```python
from build123d import *

# Parameters (mm, degrees)
F1_DEPTH = 304.8
F2_SIZE  = 50.79999
F3_SIZE  = 50.79999


# Not quite as in the source:
# - a fillet or chamfer is up to 0.001 mm smaller than in the source, because OpenCascade refuses the exact size


with BuildPart() as f1:
    # F0 (on Front) → F1 (new body, symmetric)
    with BuildSketch(Plane.XZ):
        Polygon((76.2, 3.175), (76.2, 0), (127, 0), (127, 50.8), (123.825, 50.8), (123.825, 3.175), align=None)
    extrude(amount=F1_DEPTH, both=True)

    # F2 (size 50.8 in the source; OpenCascade refuses exactly that, so slightly less here)
    f2_edges = [f1.edges().sort_by_distance(p)[0] for p in [
        (76.2, -304.8, 1.5875),
    ]]
    chamfer(f2_edges, length=F2_SIZE)

    # F3 (size 50.8 in the source; OpenCascade refuses exactly that, so slightly less here)
    f3_edges = [f1.edges().sort_by_distance(p)[0] for p in [
        (76.2, 304.8, 1.5875),
    ]]
    chamfer(f3_edges, length=F3_SIZE)


solid = f1.part
```
Could you check a few things on this model? Use its own coordinates, in mm. A direction names the side the tool comes from. Coordinates: 2 decimals unless noted, no trailing zeros. Loops run counter-clockwise (first coordinate to the right, second up) from the corner with the lowest first, then second, coordinate; pieces in that order, holes last. Notation, with made-up numbers: M 39,-2.75 L 80,-2.75 A13 ccw 80,1.25 Z; hole C 18.25,46 d1. An arc over 180 degrees is marked long. Put each result on its own line as item: value. Start each with the question number.
(1) For faces 1 (the face through (100, -4, 3.175)), 2 (the face through (113, 290.8, 2.9)), which set-ups out of +Z, -Z, +X, -X, +Y, -Y let a thin tool reach every point of the face, with its end or its side?
(2) Suppose I cut it at C-C on x = 118. Please give me the cut outline in (y, z) (3 decimals), then the cut area to 3 significant figures.
(3) Suppose I cut it at D-D on x = 92.5. Please give me the cut outline in (y, z) (3 decimals).
(4) I need wall thicknesses on line 1 (X direction, y = 58, z = 32) (3 decimals); line 2 (Z direction, x = 82.5, y = 110) (3 decimals). Which ranges of each line are inside material? Lowest first, please. Write a range as from..to.
(5) Suppose I cut it at A-A on y = -199.5. Please give me the cut outline in (x, z) (3 decimals), then the cut area to 4 significant figures.
(6) Will these pins go through, and if not, where does the flat tip stop? P1, Ø12, axis at y = 26, z = 32.5, coming from the -X side (3 decimals); P2, Ø1, axis at x = 116, y = 76, coming from the +Z side (3 decimals).
Solutions:
1. face 1: +Z, -X, +Y, -Y
1. face 2: +Z, -Z, -X, +Y
2. outline: M -295.8,0 L 295.8,0 L 295.8,3.175 L -295.8,3.175 Z
2. area: 1,880 mm2
3. outline: M -270.3,0 L 270.3,0 L 270.3,3.175 L -270.3,3.175 Z
4. line 1: x = 123.825..127
4. line 2: z = 0..3.175
5. outline: M 76.2,0 L 127,0 L 127,50.8 L 123.825,50.8 L 123.825,3.175 L 76.2,3.175 Z
5. area: 312.5 mm2
6. P1: stops at x = 123.825
6. P2: stops at z = 3.175
